Build history of the part. All positions in model axes, mm. A direction names the side the tool comes from. Give positions to 0.01 mm unless a question says otherwise; leave off trailing zeros. Order: outer loops, then holes, each group sorted by start corner. A loop starts at its lowest first (then second) coordinate and runs counter-clockwise, first axis right, second up. Notation, with made-up numbers: (25.25, -21) - (50.25, -21) arc R28 cw to (50.25, -2) - close; hole circle Ø3 at (58, 52). An arc over 180 degrees is marked (long way). Write each question's results on one line, items separated by ' | '. Start each with the question number.
1) Cut at B-B on x = 39. List the corners of the cut face in (y, z).
2) Two-plate mould, pull along Z, no slides. Class faces 5 (the face through (28.22, 5.95, -2.39)), 6 (the face through (26, -9.5, 0)), 7 (the face through (9, -3, -2.5)): +Z half, -Z half, draft (parallel to the pull), parting line (faces both ways), or undercut.
3) Tool access for faces 1 (the face through (4.194, 4.407, -5.035)), 2 (the face through (4.194, 4.407, 5.035)), 3 (the face through (18, 0, 7.5)), 4 (the face through (39, 2.5, 5)): list every direction of +Z, -Z, +X, -X, +Y, -Y with a clear straight run to the whole face (end or side of a thin tool).
4) Drop flat-ended pins along their axis: pin 1 Ø2 at (x, y) = (22, 4) entering from -Z; pin 2 Ø1.5 at (y, z) = (1.5, 7) entering from +X; pin 3 Ø4 at (x, y) = (8, 1.5) entering from -Z. Give the stop position or say it passes through.
5) Cut at C-C on y = -0.75. List the corners of the cut face in (x, z).
6) Drill centre lines: line 1 along X through (y, z) = (2.75, -5.75); line 2 along X through (y, z) = (-4, 4.75); line 3 along Y through (x, z) = (41, -4.75). Where is each one in solid material? Low to high. Write a range as from..to.
7) Cut at A-A on z = 0. List the corners of the cut face in (x, y), plus the area to 3 significant figures.
8) Cut at D-D on y = 8. List the corners of the cut face in (x, z).
from build123d import *

# Parameters (mm, degrees)
BOSS_EXTRUDE1_DEPTH        = 7.5
CORTAR_EXTRUIR1_START      = 7.5
SKETCH1_3_R                = 6.52
CORTAR_EXTRUIR1_DEPTH      = 5
CORTAR_EXTRUIR2_START      = -7.5
SKETCH1_5_R                = 6.52
CORTAR_EXTRUIR2_DEPTH      = 5
BOSS_EXTRUDE3_DEPTH        = 9.5
BOSS_EXTRUDE3_DEPTH_BACK   = 9.5
SKETCH2_R                  = 14.04
SKETCH2_R_2                = 4.25
CORTAR_EXTRUIR3_START      = -9.5
SKETCH2_4_R                = 11.04
CORTAR_EXTRUIR3_DEPTH      = 7
CORTAR_EXTRUIR4_START      = 2.5
SKETCH2_5_R                = 11.04
CORTAR_EXTRUIR4_DEPTH      = 7
CORTAR_EXTRUIR5_DEPTH      = 56.683150055
CORTAR_EXTRUIR5_DEPTH_BACK = 56.683150055
SKETCH2_6_R                = 4.25
FILLET1_R                  = 5
FILLET2_R                  = 10


with BuildPart() as part:
    # Sketch1 → Boss-Extrude1 (new, symmetric)
    with BuildSketch(Plane.XY):
        with BuildLine():
            ThreePointArc((6.75, 0), (9, 2.25), (11.25, 0))
            Line((11.25, 0), (15.52, 0))
            ThreePointArc((15.52, 0), (9, 6.52), (2.48, 0))
            Line((2.48, 0), (6.75, 0))
        make_face()
        with BuildLine():
            Line((15.52, 0), (11.25, 0))
            ThreePointArc((11.25, 0), (9, -2.25), (6.75, 0))
            Line((6.75, 0), (2.48, 0))
            ThreePointArc((2.48, 0), (9, -6.52), (15.52, 0))
        make_face()
        with BuildLine():
            ThreePointArc((2.48, 0), (9, 6.52), (15.52, 0))
            Line((15.52, 0), (39, 0))
            Line((39, 0), (39, 9.5))
            Line((39, 9.5), (0, 9.5))
            Line((0, 9.5), (0, 0))
            Line((0, 0), (2.48, 0))
        make_face()
        with BuildLine():
            Line((39, 0), (15.52, 0))
            ThreePointArc((15.52, 0), (9, -6.52), (2.48, 0))
            Line((2.48, 0), (0, 0))
            Line((0, 0), (0, -9.5))
            Line((0, -9.5), (39, -9.5))
            Line((39, -9.5), (39, 0))
        make_face()
    extrude(amount=BOSS_EXTRUDE1_DEPTH, both=True)

    # Sketch1<3> → Cortar-Extruir1 (cut)
    with BuildSketch(Plane.XY.offset(CORTAR_EXTRUIR1_START)):
        with Locations((9, 0)):
            Circle(SKETCH1_3_R)
    extrude(amount=-CORTAR_EXTRUIR1_DEPTH, mode=Mode.SUBTRACT)

    # Sketch1<5> → Cortar-Extruir2 (cut)
    with BuildSketch(Plane.XY.offset(CORTAR_EXTRUIR2_START)):
        with Locations((9, 0)):
            Circle(SKETCH1_5_R)
    extrude(amount=CORTAR_EXTRUIR2_DEPTH, mode=Mode.SUBTRACT)

    # Sketch2 → Boss-Extrude3 (add, two sides: drawn at the far end of the back side and taken through both)
    with BuildSketch(Plane(origin=(0, 0, 0), x_dir=(1, 0, 0), z_dir=(0, 1, 0)).offset(-BOSS_EXTRUDE3_DEPTH_BACK)):
        with Locations((39, 0)):
            Circle(SKETCH2_R)
        with Locations((39, 0)):
            Circle(SKETCH2_R_2, mode=Mode.SUBTRACT)
    extrude(amount=BOSS_EXTRUDE3_DEPTH + BOSS_EXTRUDE3_DEPTH_BACK)

    # Sketch2<4> → Cortar-Extruir3 (cut)
    with BuildSketch(Plane(origin=(0, 0, 0), x_dir=(1, 0, 0), z_dir=(0, 1, 0)).offset(CORTAR_EXTRUIR3_START)):
        with Locations(Location((39, 0, 0), (0, 0, 270))):
            Circle(SKETCH2_4_R)
    extrude(amount=CORTAR_EXTRUIR3_DEPTH, mode=Mode.SUBTRACT)

    # Sketch2<5> → Cortar-Extruir4 (cut)
    with BuildSketch(Plane(origin=(0, 0, 0), x_dir=(1, 0, 0), z_dir=(0, 1, 0)).offset(CORTAR_EXTRUIR4_START)):
        with Locations(Location((39, 0, 0), (0, 0, 270))):
            Circle(SKETCH2_5_R)
    extrude(amount=CORTAR_EXTRUIR4_DEPTH, mode=Mode.SUBTRACT)

    # Sketch2<6> → Cortar-Extruir5 (cut, two sides: drawn at the far end of the back side and taken through both)
    with BuildSketch(Plane(origin=(0, 0, 0), x_dir=(1, 0, 0), z_dir=(0, 1, 0)).offset(-CORTAR_EXTRUIR5_DEPTH_BACK)):
        with Locations(Location((39, 0, 0), (0, 0, 270))):
            Circle(SKETCH2_6_R)
    extrude(amount=CORTAR_EXTRUIR5_DEPTH + CORTAR_EXTRUIR5_DEPTH_BACK, mode=Mode.SUBTRACT)

    # Fillet1
    fillet1_edges = [part.edges().sort_by_distance(p)[0] for p in [
        (27.13106576, 0, -7.5),
        (27.13106576, 0, 7.5),
    ]]
    fillet(fillet1_edges, radius=FILLET1_R)

    # Fillet2
    # the kernel refuses this fillet: 10 mm, written as the material it takes off along each edge
    with BuildSketch(Plane(origin=(0, -9.5, 32.5), x_dir=(1, 0, 0), z_dir=(0, 0, -1)), Plane(origin=(0, 9.5, 32.5), x_dir=(0, -1, 0), z_dir=(0, 0, -1))) as fillet2_piece_1:
        with BuildLine():
            CenterArc((FILLET2_R, -FILLET2_R), FILLET2_R, 90, 90)
            Line((0, -FILLET2_R), (0, 0))
            Line((0, 0), (FILLET2_R, 0))
        make_face()
    extrude(amount=65, mode=Mode.SUBTRACT)


solid = part.part
Results:
1) outline: (-9.5, -14.04) - (9.5, -14.04) - (9.5, -11.04) - (2.5, -11.04) - (2.5, -4.25) - (-2.5, -4.25) - (-2.5, -11.04) - (-9.5, -11.04) - close; (-9.5, 11.04) - (-2.5, 11.04) - (-2.5, 4.25) - (2.5, 4.25) - (2.5, 11.04) - (9.5, 11.04) - (9.5, 14.04) - (-9.5, 14.04) - close
2) face 5: undercut | face 6: draft | face 7: -Z half
3) face 1: -Z | face 2: +Z | face 3: +Z, -X, +Y, -Y | face 4: +Y
4) pin 1: z = -7.5 | pin 2: x = 51.57 | pin 3: z = -2.5
5) outline: (0.08, -7.5) - (2.52, -7.5) - (2.52, -2.5) - (6.88, -2.5) - (6.88, 2.5) - (2.52, 2.5) - (2.52, 7.5) - (0.08, 7.5) - close; (11.12, -2.5) - (15.48, -2.5) - (15.48, -7.5) - (24.64, -7.5) arc R5 cw to (28.41, -9.22) arc R14.04 ccw (long way) to (28.41, 9.22) arc R5 cw to (24.64, 7.5) - (15.48, 7.5) - (15.48, 2.5) - (11.12, 2.5) - close; hole circle Ø8.5 at (39, 0)
6) line 1: 0.54..3.09, 14.91..29.58, 48.42..51.81 | line 2: 1.07..3.85, 14.15..29.03, 48.97..52.21 | line 3: -2.5..2.5
7) outline: (0.01, 0) arc R10 ccw to (10, -9.5) - (27.96, -9.5) - (27.96, -2.5) - (34.75, -2.5) - (34.75, 2.5) - (27.96, 2.5) - (27.96, 9.5) - (10, 9.5) arc R10 ccw to start; (43.25, -2.5) - (50.04, -2.5) - (50.04, -9.5) - (53.04, -9.5) - (53.04, 9.5) - (50.04, 9.5) - (50.04, 2.5) - (43.25, 2.5) - close; hole circle Ø4.5 at (9, 0) | area: 597 mm^2
8) outline: (4.73, -7.5) - (24.64, -7.5) arc R5 cw to (28.41, -9.22) arc R14.04 ccw (long way) to (28.41, 9.22) arc R5 cw to (24.64, 7.5) - (4.73, 7.5) - close; hole circle Ø22.08 at (39, 0)
